Work out the finished part from the listing and answer in its coordinate system (mm). A direction names the side the tool comes from. Give positions to 0.01 mm unless a question says otherwise; leave off trailing zeros. Write each loop counter-clockwise with the first axis right and the second up, starting at its lowest first coordinate (ties: lowest second). Pieces come first, ordered by that corner, then holes.
1) Find section A-A (y = -16). Determine the outline of the cut face in (x, z), plus the area to 3 significant figures.
2) Straight lines are drawn through the part: probe 1 along X at (y, z) = (-31.5, 1.5); probe 2 along Y at (x, z) = (-57, -4.5). For each, find the intervals that lie inside material, in ascending order.
3) Find section C-C (x = -23.5). Determine the outline of the cut face in (y, z), plus the area to 3 significant figures.
4) A tool of negligible diameter and unlimited length cuts with its end or side. For faces 4 (the face through (-61.777, -36.587, 6.073)), 5 (the face through (-61.777, -17.34, 23.697)), 6 (the face through (-61.15, -22, -2)), from which of +Z, -Z, +X, -X, +Y, -Y can it reach the whole face along a straight path? Write none if from no direction.
5) Find section B-B (z = 21). Determine the outline of the cut face in (x, y).
6) Find section D-D (z = -7). Determine the outline of the cut face in (x, y), plus the area to 3 significant figures.
7) Determine the mould class of faces 1 (the face through (61.777, -36.587, 6.073)), 2 (the face through (61.15, -22, -2)), 3 (the face through (-61.777, -28.303, 28.918)) for opening direction Y: pulls with the +Y half, pulls with the -Y half, needs draft (parallel to the pull), parting line crosses it, or undercut.
8) Given pin 1 Ø1.5 at (x, z) = (5, -15) entering from -Y; pin 2 Ø0.9 at (x, y) = (-14.5, -1.5) entering from +Z; pin 3 Ø5 at (y, z) = (-34.57, -19.05) entering from -X; pin 4 Ø4 at (x, y) = (-25.5, -4.5) entering from -Z, each flat-ended and moving along its own axis, determine where each tip first touches the part or whether it passes through.
```python
from build123d import *

# Parameters (mm, degrees)
F0_W     = 122.301
F0_H     = 50.8
F1_DEPTH = 1.27
F2_W     = 1.27
F2_H     = 50.8
F2_R     = 2.159
F3_DEPTH = 1.27
F5_R     = 1.016


with BuildPart() as f1:
    # F0 (on Front) → F1 (new body)
    with BuildSketch(Plane.XZ):
        Rectangle(F0_W, F0_H)
    extrude(amount=F1_DEPTH)

    # F2 (on face) → F3 (join)
    with BuildSketch(Plane.YZ.offset(61.1505)):
        with Locations((-0.635, 0)):
            Rectangle(F2_W, F2_H)
        with BuildLine():
            Line((-34.5694, -25.4), (-1.27, -25.4))
            Line((-1.27, -25.4), (-1.27, 25.4))
            Line((-1.27, 25.4), (-3.048, 25.4))
            ThreePointArc((-3.048, 25.4), (-12.9705871442, 30.9789160504), (-23.835727376, 34.3746144578))
            ThreePointArc((-23.835727376, 34.3746144578), (-25.1069267062, 34.6143527598), (-26.3834586647, 34.8238482236))
            ThreePointArc((-26.3834586647, 34.8238482236), (-30.4019207613, 33.2281345448), (-32.4672506211, 29.4296147888))
            Line((-32.4672506211, 29.4296147888), (-40.8229292316, -17.9473340718))
            ThreePointArc((-40.8229292316, -17.9473340718), (-39.4337822138, -23.1317013215), (-34.5694, -25.4))
        make_face()
        with Locations((-34.5694, -19.05)):
            Circle(F2_R, mode=Mode.SUBTRACT)
        with BuildLine():
            ThreePointArc((-26.4055731828, 26.3286980436), (-28.291565828, 28.9678233876), (-25.4317316722, 30.4986073176))
            ThreePointArc((-25.4317316722, 30.4986073176), (-15.6793239493, 27.7117353818), (-6.7247772333, 22.9481018219))
            ThreePointArc((-6.7247772333, 22.9481018219), (-5.617517065, 20.1630344292), (-8.3603573385, 18.954956329))
            ThreePointArc((-8.3603573385, 18.954956329), (-8.8006503817, 19.1767894333), (-9.1791381358, 19.4927244109))
            ThreePointArc((-9.1791381358, 19.4927244109), (-17.4611225454, 23.7454080866), (-26.4055731828, 26.3286980436))
        make_face(mode=Mode.SUBTRACT)
    extrude(amount=F3_DEPTH)

    # F4: F1 across plane


with BuildPart() as f1_1:
    add(f1.part)
    add(f1.part.mirror(Plane.YZ))

    # F5
    f5_edges = [f1_1.edges().sort_by_distance(p)[0] for p in [
        (-62.4205, 0, 0),
        (62.4205, 0, 0),
        (61.1505, -1.27, 0),
        (-61.1505, -1.27, 0),
    ]]
    fillet(f5_edges, radius=F5_R)


solid = f1_1.part
```
Results:
1. outline: (-62.42, -25.4) - (-61.15, -25.4) - (-61.15, 23.14) - (-62.42, 23.14) - close; (-62.42, 27.84) - (-61.15, 27.84) - (-61.15, 32.18) - (-62.42, 32.18) - close; (61.15, -25.4) - (62.42, -25.4) - (62.42, 23.14) - (61.15, 23.14) - close; (61.15, 27.84) - (62.42, 27.84) - (62.42, 32.18) - (61.15, 32.18) - close
1. area: 134 mm2
2. probe 1: x = -62.42 to -61.15, 61.15 to 62.42
2. probe 2: y = -1.27 to 0
3. outline: (-1.27, -25.4) - (0, -25.4) - (0, 25.4) - (-1.27, 25.4) - close
3. area: 64.5 mm2
4. face 4: +Z, +X, -X, -Y
4. face 5: +X, -X
4. face 6: +Z, -Z, -Y
5. outline: (-62.42, -33.95) - (-61.15, -33.95) - (-61.15, -11.69) - (-62.42, -11.69) - close; (-62.42, -5.46) - (-61.15, -5.46) - (-61.15, -2.29) arc R1.02 cw to (-60.13, -1.27) - (60.13, -1.27) arc R1.02 cw to (61.15, -2.29) - (61.15, -5.46) - (62.42, -5.46) - (62.42, -1.02) arc R1.02 ccw to (61.4, 0) - (-61.4, 0) arc R1.02 ccw to (-62.42, -1.02) - close; (61.15, -33.95) - (62.42, -33.95) - (62.42, -11.69) - (61.15, -11.69) - close
6. outline: (-62.42, -38.89) - (-61.15, -38.89) - (-61.15, -2.29) arc R1.02 cw to (-60.13, -1.27) - (60.13, -1.27) arc R1.02 cw to (61.15, -2.29) - (61.15, -38.89) - (62.42, -38.89) - (62.42, -1.02) arc R1.02 ccw to (61.4, 0) - (-61.4, 0) arc R1.02 ccw to (-62.42, -1.02) - close
6. area: 254 mm2
7. face 1: pulls with the -Y half
7. face 2: needs draft
7. face 3: undercut
8. pin 1: stops at y = -1.27
8. pin 2: stops at z = 25.4
8. pin 3: stops at x = -62.42
8. pin 4: passes through
